```python
from build123d import *

# Parameters (mm, degrees)
KEEPOUTLAYER_W      = 186.9999816
KEEPOUTLAYER_H      = 76.9999984
EXTRUDE_1_DEPTH     = 1.6
VIAHOLELAYER_R      = 0.7499985
CUT_EXTRUDE_1_DEPTH = 2.6
SKETCH_2_W          = 5
SKETCH_2_H          = 1.6
EXTRUDE_3_DEPTH     = 2.5


with BuildPart() as part:
    # KeepOutLayer → Бобышка-Вытянуть1 (new body)
    with BuildSketch(Plane.XY):
        with Locations((93.56941662, -38.56797722)):
            Rectangle(KEEPOUTLAYER_W, KEEPOUTLAYER_H)
    extrude(amount=-EXTRUDE_1_DEPTH)

    # ViaHoleLayer → Вырез-Вытянуть1 (cut, through all)
    with BuildSketch(Plane.XY):
        with Locations((3.0693995, -73.06799966)):
            Circle(VIAHOLELAYER_R)
        with Locations((3.0693995, -4.0680005)):
            Circle(VIAHOLELAYER_R)
        with Locations((184.06940072, -73.06799966)):
            Circle(VIAHOLELAYER_R)
        with Locations((184.06940072, -4.0680005)):
            Circle(VIAHOLELAYER_R)
    extrude(amount=-CUT_EXTRUDE_1_DEPTH, mode=Mode.SUBTRACT)

    # Эскиз2 → Бобышка-Вытянуть3 (add)
    with BuildSketch(Plane(origin=(0, -0.06797802, 0), x_dir=(1, 0, 0), z_dir=(0, 1, 0))):
        with Locations((52.56942582, 0.8)):
            Rectangle(SKETCH_2_W, SKETCH_2_H)
    extrude(amount=EXTRUDE_3_DEPTH)


solid = part.part
```
Read the model definition and answer for the solid it produces. Units are mm, in the model's axes. Round coordinates to 2 decimals unless told otherwise and drop trailing zeros. Write each loop counter-clockwise with the first axis right and the second up, starting at its lowest first coordinate (ties: lowest second). Pieces come first, ordered by that corner, then holes. Notation, with made-up numbers: (-7, 55.5) -> (14, 55.5) arc R21 cw to (14, 66.5) -> close; hole circle Ø4 at (27.25, -12). An arc over 180 degrees is marked (long way). Answer in a Markdown table with one row per item. Add a question column.
1) Consider line 1 (Y direction, x = 151, z = -0.85); line 2 (X direction, y = -4.5, z = -1.2). Determine where each line is inside the solid, lowest interval first.
2) Find section A-A, the plane z = -0.35. Determine the outline of the cut face in (x, y).
3) Given P1, Ø0.8, axis at x = 33, z = -0.5, coming from the +Y side; P2, Ø0.8, axis at y = 1.5, z = -1, coming from the +X side, each flat-ended and moving along its own axis, determine where each tip first touches the part or whether it passes through.
4) Find section B-B, the plane x = 67.5. Determine the outline of the cut face in (y, z), and give its area (3 significant figures).
Findings below:
| question | item | result |
|---|---|---|
| 1 | line 1 | -77.07 to -0.07 |
| 1 | line 2 | 0.07 to 2.46, 3.68 to 183.46, 184.68 to 187.07 |
| 2 | outline | (0.07, -77.07) -> (187.07, -77.07) -> (187.07, -0.07) -> (55.07, -0.07) -> (55.07, 2.43) -> (50.07, 2.43) -> (50.07, -0.07) -> (0.07, -0.07) -> close; hole circle Ø1.5 at (3.07, -73.07); hole circle Ø1.5 at (3.07, -4.07); hole circle Ø1.5 at (184.07, -73.07); hole circle Ø1.5 at (184.07, -4.07) |
| 3 | P1 | y = -0.07 |
| 3 | P2 | x = 55.07 |
| 4 | outline | (-77.07, -1.6) -> (-0.07, -1.6) -> (-0.07, 0) -> (-77.07, 0) -> close |
| 4 | area | 123 mm² |
